The model under review builds one solid part; all positions refer to its coordinate system, in mm. A direction names the side the tool comes from. Give positions to 0.01 mm unless a question says otherwise; leave off trailing zeros. Loops run counter-clockwise (first coordinate to the right, second up) from the corner with the lowest first, then second, coordinate; pieces in that order, holes last. Notation, with made-up numbers: M 54,12 L 79,12 A9 ccw 79,25 Z; hole C -16,82 d1. An arc over 180 degrees is marked long. One line per item, written item: value. Start each with the question number.
Q1. To check wall thickness, follow line 1 along X through (y, z) = (-24.75, 63.5); line 2 along Y through (x, z) = (6.5, -70); line 3 along X through (y, z) = (14.5, 31). State the ranges of each line that lie inside material, in increasing order. Write a range as from..to.
Q2. For pin 1 (6.5 mm diameter, centred on x = 0, z = 63.5, fed in from -Y), flat-tipped, find the tip position at first contact; note if it passes through.
Q3. For faces 4 (the face through (-0.269, 24.148, 61.448)), 5 (the face through (-10.16, 0, 1)), list the 3-axis set-ups (+Z, -Z, +X, -X, +Y, -Y) from which the entire face can be reached by the end or side of a thin tool; tool diameter is ignored.
Q4. We need section B-B on x = -7.25. Write out the cut boundary in (y, z), plus the area to 3 significant figures.
Q5. We need section A-A on y = 0. Write out the cut boundary in (x, z), plus the area to 3 significant figures.
Q6. We need section D-D on z = 63.5. Write out the cut boundary in (x, y).
Q7. We need section C-C on z = -16.5. Write out the cut boundary in (x, y), plus the area to 3 significant figures.
Q8. Mouldability with a two-part tool opening along Z and no side actions: class faces 1 (the face through (-0.269, -24.112, 61.448)), 2 (the face through (10.16, 0, 1)), 3 (the face through (-10.4, 2, 76.2)) as released by +Z, released by -Z, zero draft, split by the parting line, or undercut.
```python
from build123d import *

# Parameters (mm, degrees)
SKETCH1_W           = 25.4
SKETCH1_H           = 50.8
SKETCH1_W_2         = 20.32
SKETCH1_H_2         = 45.72
EXTRUDE_THIN1_DEPTH = 76.2
SKETCH2_R           = 2.0701
CUT_EXTRUDE1_DEPTH  = 51.8
LPATTERN1_COUNT     = 7
LPATTERN1_PITCH     = 25.4
SKETCH3_R           = 2.4892
CUT_EXTRUDE2_DEPTH  = 26.4


with BuildPart() as part:
    # Sketch1 → Extrude-Thin1 (new body, symmetric)
    with BuildSketch(Plane.XY):
        Rectangle(SKETCH1_W, SKETCH1_H)
        Rectangle(SKETCH1_W_2, SKETCH1_H_2, mode=Mode.SUBTRACT)
    extrude(amount=EXTRUDE_THIN1_DEPTH, both=True)

    # Sketch2 → Cut-Extrude1 (cut, through all)
    with BuildSketch(Plane(origin=(0, 25.4, 0), x_dir=(1, 0, 0), z_dir=(0, 1, 0))):
        with Locations((0, -63.5)):
            Circle(SKETCH2_R)
    cut_extrude1 = extrude(amount=-CUT_EXTRUDE1_DEPTH, mode=Mode.SUBTRACT)

    # LPattern1: Cut-Extrude1 ×7
    with Locations(*[(0, 0, -i * LPATTERN1_PITCH) for i in range(1, LPATTERN1_COUNT)]):
        add(cut_extrude1, mode=Mode.SUBTRACT)

    # Sketch3 → Cut-Extrude2 (cut, through all)
    with BuildSketch(Plane(origin=(12.7, 0, 0), x_dir=(0, 0, -1), z_dir=(1, 0, 0))):
        with Locations((61.9125, 0)):
            Circle(SKETCH3_R)
    extrude(amount=-CUT_EXTRUDE2_DEPTH, mode=Mode.SUBTRACT)


solid = part.part
```
Solved:
1. line 1: -12.7..-2.07, 2.07..12.7
1. line 2: -25.4..-22.86, 22.86..25.4
1. line 3: -12.7..-10.16, 10.16..12.7
2. pin 1: y = -25.4
3. face 4: +Y, -Y
3. face 5: +Z, -Z
4. outline: M -25.4,-76.2 L -22.86,-76.2 L -22.86,76.2 L -25.4,76.2 Z; M 22.86,-76.2 L 25.4,-76.2 L 25.4,76.2 L 22.86,76.2 Z
4. area: 774 mm2
5. outline: M -12.7,-76.2 L -10.16,-76.2 L -10.16,-64.4 L -12.7,-64.4 Z; M -12.7,-59.42 L -10.16,-59.42 L -10.16,76.2 L -12.7,76.2 Z; M 10.16,-76.2 L 12.7,-76.2 L 12.7,-64.4 L 10.16,-64.4 Z; M 10.16,-59.42 L 12.7,-59.42 L 12.7,76.2 L 10.16,76.2 Z
5. area: 749 mm2
6. outline: M -12.7,-25.4 L -2.07,-25.4 L -2.07,-22.86 L -10.16,-22.86 L -10.16,22.86 L -2.07,22.86 L -2.07,25.4 L -12.7,25.4 Z; M 2.07,-25.4 L 12.7,-25.4 L 12.7,25.4 L 2.07,25.4 L 2.07,22.86 L 10.16,22.86 L 10.16,-22.86 L 2.07,-22.86 Z
7. outline: M -12.7,-25.4 L 12.7,-25.4 L 12.7,25.4 L -12.7,25.4 Z; hole M -10.16,-22.86 L 10.16,-22.86 L 10.16,22.86 L -10.16,22.86 Z
7. area: 361 mm2
8. face 1: undercut
8. face 2: zero draft
8. face 3: released by +Z
